Geometry check sheet. Reference: the model listing, model coordinates, mm. Face numbers are marked on the shaded views. A direction names the side the tool comes from. Round coordinates to 2 decimals unless told otherwise and drop trailing zeros. Order: outer loops, then holes, each group sorted by start corner. A loop starts at its lowest first (then second) coordinate and runs counter-clockwise, first axis right, second up.
(1) Sectioned sample at A-A (y = 5.5). Record the boundary of the cut face in (x, z).
(2) Sectioned sample at B-B (z = 13). Record the boundary of the cut face in (x, y), plus the area to 3 significant figures.
(3) Set-up check for the marked faces 1, 2, 3 and 4: record each of +Z, -Z, +X, -X, +Y, -Y from which the full face is reachable in a straight line by a thin tool's end or side.
(4) Sectioned sample at C-C (x = 29.5). Record the boundary of the cut face in (y, z).
(5) Go/stop test with flat-tipped pins: pin 1 (12 mm diameter, centred on x = 9.5, z = -20, fed in from +Y); pin 2 (5 mm diameter, centred on y = -25.5, z = -10.5, fed in from +X); pin 3 (2.5 mm diameter, centred on y = -26.5, z = 26.5, fed in from +X). Record where each tip stops, or that it passes through.
(6) Sectioned sample at D-D (y = 32). Record the boundary of the cut face in (x, z).
(7) Material ranges on line 1 along Y through (x, z) = (1, 8); line 2 along X through (y, z) = (-24, -28.5), recorded low to high.
from build123d import *

# Parameters (mm, degrees)
F0_R      = 38.1
F1_DEPTH  = 25.4
F2_R      = 38.1
F3_DEPTH  = 25.4
F4_R      = 38.1
F5_DEPTH  = 25.4
F6_R      = 38.1
F7_DEPTH  = 25.4
F8_R      = 38.1
F9_DEPTH  = 25.4
F10_R     = 38.1
F11_DEPTH = 25.4


with BuildPart() as f1:
    # F0 (on Front) → F1 (new body)
    with BuildSketch(Plane.XZ):
        Circle(F0_R)
    extrude(amount=F1_DEPTH)

    # F2 (on Top) → F3 (join)
    with BuildSketch(Plane.XY):
        Circle(F2_R)
    extrude(amount=F3_DEPTH)

    # F4 (on Right) → F5 (join)
    with BuildSketch(Plane.YZ):
        Circle(F4_R)
    extrude(amount=F5_DEPTH)

    # F6 (on Top) → F7 (join)
    with BuildSketch(Plane.XY):
        Circle(F6_R)
    extrude(amount=-F7_DEPTH)

    # F8 (on Front) → F9 (join)
    with BuildSketch(Plane.XZ):
        Circle(F8_R)
    extrude(amount=-F9_DEPTH)

    # F10 (on Right) → F11 (join)
    with BuildSketch(Plane.YZ):
        Circle(F10_R)
    extrude(amount=-F11_DEPTH)


solid = f1.part
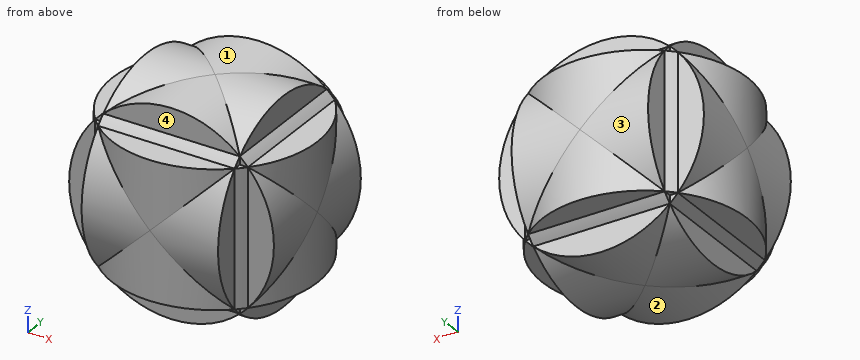
Answer below:
1. outline: (-37.7, -25.4) - (-28.4, -25.4) arc R38.1 ccw to (-25.4, -28.4) - (-25.4, -37.7) - (-5.5, -37.7) arc R38.1 ccw to (5.5, -37.7) - (25.4, -37.7) - (25.4, -28.4) arc R38.1 ccw to (28.4, -25.4) - (37.7, -25.4) - (37.7, -5.5) arc R38.1 ccw to (37.7, 5.5) - (37.7, 25.4) - (28.4, 25.4) arc R38.1 ccw to (25.4, 28.4) - (25.4, 37.7) - (5.5, 37.7) arc R38.1 ccw to (-5.5, 37.7) - (-25.4, 37.7) - (-25.4, 28.4) arc R38.1 ccw to (-28.4, 25.4) - (-37.7, 25.4) - (-37.7, 5.5) arc R38.1 ccw to (-37.7, -5.5) - close
2. outline: (-35.81, -25.4) - (-28.4, -25.4) arc R38.1 ccw to (-25.4, -28.4) - (-25.4, -35.81) - (-13, -35.81) arc R38.1 ccw to (13, -35.81) - (25.4, -35.81) - (25.4, -28.4) arc R38.1 ccw to (28.4, -25.4) - (35.81, -25.4) - (35.81, -13) arc R38.1 ccw to (35.81, 13) - (35.81, 25.4) - (28.4, 25.4) arc R38.1 ccw to (25.4, 28.4) - (25.4, 35.81) - (13, 35.81) arc R38.1 ccw to (-13, 35.81) - (-25.4, 35.81) - (-25.4, 28.4) arc R38.1 ccw to (-28.4, 25.4) - (-35.81, 25.4) - (-35.81, 13) arc R38.1 ccw to (-35.81, -13) - close
2. area: 4,870 mm2
3. face 1: +Z, +Y
3. face 2: -Z, -Y
3. face 3: -X, +Y
3. face 4: +Z, +X, -X, -Y
4. outline: (-25.4, -24.11) - (-24.11, -24.11) - (-24.11, -25.4) - (24.11, -25.4) - (24.11, -24.11) - (25.4, -24.11) - (25.4, 24.11) - (24.11, 24.11) - (24.11, 25.4) - (-24.11, 25.4) - (-24.11, 24.11) - (-25.4, 24.11) - close
5. pin 1: stops at y = 37.94
5. pin 2: stops at x = 37.25
5. pin 3: stops at x = 27.94
6. outline: (-25.4, -20.68) - (-20.68, -20.68) - (-20.68, -25.4) - (20.68, -25.4) - (20.68, -20.68) - (25.4, -20.68) - (25.4, 20.68) - (20.68, 20.68) - (20.68, 25.4) - (-20.68, 25.4) - (-20.68, 20.68) - (-25.4, 20.68) - close
7. line 1: y = -38.09 to 38.09
7. line 2: x = -25.4 to 25.4
